Autodesk Inventor part; units mm, degrees
ref_plane "作業平面1" through (97.746748, 12.158256, 0) normal (0.9923528, 0.1234341, 0) x (-0.1234341, 0.9923528, 0)
ref_plane "YZ Plane" through (0, 0, 0) normal (1, 0, 0) x (0, 1, 0)
ref_plane "XZ Plane" through (0, 0, 0) normal (0, 1, 0) x (-1, 0, 0)
sketch "スケッチ1" plane through (0, 0, 0) normal (0, 0, 1) x (1, 0, 0)
  circle A0 centre (0, 0) radius 98.5
  circle A1 centre (0, 0) radius 86.5
  circle A2 centre (86.5, 0) radius 4
  circle A3 centre (86.5, 0) radius 7
  line L0 (0, 0) -> (98.5, 0)
  circle A4 centre (0, 0) radius 93.5
  line L1 (0, 0) -> (97.003564, 17.104346)
  line L2 (0, 0) -> (98.17694, -7.971098)
  line L3 (86.5, 0) -> (83, 6.062178)
  line L4 (86.5, 0) -> (83, -6.062178)
  line L5 (97.746748, 12.158256) -> (0, 0)
  point P0 (84.5, -3.464102)
  point P1 (83, -6.062178)
  point P2 (86.216763, -6.994267)
  point P3 (86.216298, -7)
  point P4 (92.079525, 16.236105)
  point P5 (93.5, 0)
  point P6 (84.5, 3.464102)
  dimension "d1" = 173
  dimension "d3" = 14
  dimension "d0" = 197
  dimension "d2" = 8
  dimension "d4" = 187
  dimension "d5" = 10
  dimension "d6" = 60
  dimension "d11" = 5
  dimension "d20" = 7.09
sketch "スケッチ1 outline for 押し出し1" plane through (0, 0, 0) normal (0, 0, 1) x (1, 0, 0)
  arc A0 (84.5, 3.464102) -> (84.5, -3.464102) centre (86.5, 0) cw
  line L0 (83, 6.062178) -> (84.5, 3.464102)
  arc A1 (93.5, 0) -> (83, 6.062178) centre (86.5, 0) ccw
  arc A2 (92.079525, 16.236105) -> (93.5, 0) centre (0, 0) cw
  line L1 (97.003564, 17.104346) -> (92.079525, 16.236105)
  arc A3 (98.17694, -7.971098) -> (97.003564, 17.104346) centre (0, 0) ccw
  line L2 (86.216298, -7) -> (98.17694, -7.971098)
  arc A4 (86.216763, -6.994267) -> (86.216298, -7) centre (-0.000023, 0.000002) cw
  arc A5 (83, -6.062178) -> (86.216763, -6.994267) centre (86.5, 0) ccw
  line L3 (84.5, -3.464102) -> (83, -6.062178)
extrude "押し出し1" add sketch "スケッチ1 outline for 押し出し1" along normal blind 10
ref_plane "作業平面1" through (97.746748, 12.158256, 0) normal (0.9923528, 0.1234341, 0) x (-0.1234341, 0.9923528, 0)
sketch "スケッチ2" plane through (97.746748, 12.158256, 0) normal (0.9923528, 0.1234341, 0) x (-0.1234341, 0.9923528, 0)
  line L0 (5, 10) -> (-20.028521, 10)
  point P0 (0, 0)
  point P1 (0, 5)
  dimension "d12" = 5
hole "穴1" at (97.746748, 12.158256, 5) direction (-0.9923528, -0.1234341, 0) diameter 3.4 end through all
fillet "フィレット1" radius 1 7 edges at (83, -6.0622, 5) (84.5, -3.4641, 5) (84.5, 3.4641, 5) (83, 6.0622, 5) (93.5, 0, 5) (92.0795, 16.2361, 5) (97.0036, 17.1043, 5)
fillet "フィレット2" radius 5 1 edges at (98.1769, -7.9711, 5)
properties part number "TH22_3DP_cover_fixer_sn" material "ABS プラスチック"
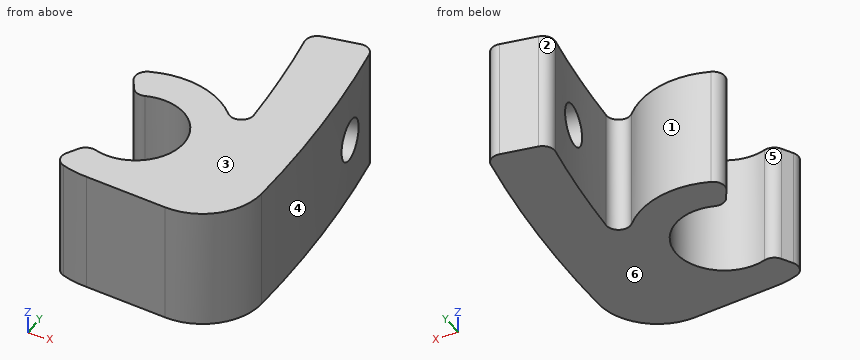
Model file for the job. Use its own axes, mm. Face numbers are marked on the shaded views. A direction names the side the tool comes from. Give positions to 0.01 mm unless a question says otherwise; leave off trailing zeros. Write each loop counter-clockwise with the first axis right and the second up, starting at its lowest first coordinate (ties: lowest second). Pieces come first, ordered by that corner, then holes. Notation, with made-up numbers: M -3.75,-14.5 L 49.25,-14.5 A25 cw 49.25,13.5 Z; hole C 11.5,23 d2. An arc over 180 degrees is marked long. Use a Markdown table: item, result.
1) Cut at D-D (x = 91). List the corners of the cut face in (y, z).
Responses:
| item | result |
|---|---|
| outline | M -7.39,0 L 5.36,0 L 5.36,10 L -7.39,10 Z |
2) Cut at C-C (y = 0). List the corners of the cut face in (x, z).
Responses:
| item | result |
|---|---|
| outline | M 90.5,0 L 98.5,0 L 98.5,10 L 90.5,10 Z |
3) Tool access for the marked faces 4, 5 and 6: list every direction of +Z, -Z, +X, -X, +Y, -Y with a clear straight run to the whole face (end or side of a thin tool).
Responses:
| item | result |
|---|---|
| face 4 | +Z, -Z, +X |
| face 5 | +Z, -Z |
| face 6 | -Z, +X, -X, +Y, -Y |
4) Cut at A-A (x = 86.5). List the corners of the cut face in (y, z).
Responses:
| item | result |
|---|---|
| outline | M -7.02,0 L -4,0 L -4,10 L -7.02,10 Z; M 4,0 L 7,0 L 7,10 L 4,10 Z |
5) Cut at B-B (y = 6). List the corners of the cut face in (x, z), and give its area (3 significant figures).
Responses:
| item | result |
|---|---|
| outline | M 83.48,0 L 90.11,0 L 90.11,10 L 83.48,10 Z; M 93.31,0 L 98.32,0 L 98.32,10 L 93.31,10 Z |
| area | 116 mm2 |
6) Pull direction X, two halves, no side cores. Call the marked faces 1, 2 and 3: +X half, -X half, draft (parallel to the pull), parting line (faces both ways), or undercut.
Responses:
| item | result |
|---|---|
| face 1 | undercut |
| face 2 | -X half |
| face 3 | draft |
7) Pin check, flat tips, straight feed: pin 1 (6 mm diameter, centred on x = 87.5, z = 3.5, fed in from +Y); pin 2 (5 mm diameter, centred on y = 7.5, z = 7, fed in from +X); pin 3 (2 mm diameter, centred on y = 0.5, z = 5.5, fed in from -X). Stop position of each tip, or through.
Responses:
| item | result |
|---|---|
| pin 1 | stops at y = 7 |
| pin 2 | stops at x = 98.37 |
| pin 3 | stops at x = 90.21 |
8) Drill centre lines: line 1 (X direction, y = 0, z = 7.25); line 2 (Y direction, x = 86.5, z = 7.25); line 3 (Y direction, x = 95.25, z = 6.5). Where is each one in solid material? Low to high. Write a range as from..to.
Responses:
| item | result |
|---|---|
| line 1 | x = 90.5..98.5 |
| line 2 | y = -7.02..-4, 4..7 |
| line 3 | y = -7.24..11.04, 12.65..16.8 |
